Read the model definition and answer for the solid it produces. Units are mm, in the model's axes. Round coordinates to 2 decimals unless told otherwise and drop trailing zeros. Order: outer loops, then holes, each group sorted by start corner. A loop starts at its lowest first (then second) coordinate and runs counter-clockwise, first axis right, second up. Notation, with made-up numbers: (-33, -9.5) -> (22, -9.5) arc R22 ccw to (22, 14.5) -> close; hole circle Ø3 at (16, 17.25). An arc over 180 degrees is marked (long way). One line per item, written item: value. Start each with the question number.
1. Flat-ended cylindrical pins translate along their axes: pin 1 Ø1.5 at (x, y) = (-18.5, 1.5) entering from +Z; pin 2 Ø1 at (x, y) = (-9.5, 1.5) entering from -Z. Find the tip coordinate at first contact, or state that the pin passes through.
2. Section C-C (y = 1.55) is taken. Give the vertices of the cut face in (x, z).
3. Consider line 1 (Z direction, x = 0, y = 1.5); line 2 (Z direction, x = -11.5, y = 2.9); line 3 (X direction, y = 1.1, z = 6). Determine where each line is inside the solid, lowest interval first.
4. Section B-B (x = 0) is taken. Give the vertices of the cut face in (y, z), then the cut area to 3 significant figures.
5. Section A-A (z = 0) is taken. Give the vertices of the cut face in (x, y).
6. The mould has two halves that part along X. Classify faces 1 (the face through (12, 3, 6)), 2 (the face through (11.99, 1.51, 0.53)), 3 (the face through (13.38, 1.49, 25.73)): released by +X, released by -X, zero draft, split by the parting line, or undercut.
from build123d import *

# Parameters (mm, degrees)
SKETCH1_R          = 29
EXTRUDE1_DEPTH     = 3
SKETCH2_R          = 12
CUT_EXTRUDE1_DEPTH = 4
CHAMFER1_SIZE      = 0.5
CHAMFER2_SIZE      = 1


with BuildPart() as part:
    # Sketch1 → Extrude1 (new body)
    with BuildSketch(Plane(origin=(0, 0, 0), x_dir=(1, 0, 0), z_dir=(0, 1, 0))):
        Circle(SKETCH1_R)
    extrude(amount=EXTRUDE1_DEPTH)

    # Sketch2 → Cut-Extrude1 (cut, through all)
    with BuildSketch(Plane(origin=(0, 3, 0), x_dir=(-1, 0, 0), z_dir=(0, 1, 0))):
        Circle(SKETCH2_R)
    extrude(amount=-CUT_EXTRUDE1_DEPTH, mode=Mode.SUBTRACT)

    # Chamfer1
    chamfer1_edges = [part.edges().sort_by_distance(p)[0] for p in [
        (-29, 0, 0),
        (-29, 3, 0),
    ]]
    chamfer(chamfer1_edges, length=CHAMFER1_SIZE)

    # Chamfer2
    chamfer2_edges = [part.edges().sort_by_distance(p)[0] for p in [
        (12, 0, 0),
        (12, 3, 0),
    ]]
    chamfer(chamfer2_edges, length=CHAMFER2_SIZE)


solid = part.part
Answer:
1. pin 1: z = 22.93
1. pin 2: z = -27.57
2. outline: circle Ø58 at (0, 0); hole circle Ø24 at (0, 0)
3. line 1: -29 to -12, 12 to 29
3. line 2: -26.19 to -5.84, 5.84 to 26.19
3. line 3: -28.37 to -10.39, 10.39 to 28.37
4. outline: (0, -28.5) -> (0.5, -29) -> (2.5, -29) -> (3, -28.5) -> (3, -13) -> (2, -12) -> (1, -12) -> (0, -13) -> close; (0, 13) -> (1, 12) -> (2, 12) -> (3, 13) -> (3, 28.5) -> (2.5, 29) -> (0.5, 29) -> (0, 28.5) -> close
4. area: 99.5 mm^2
5. outline: (-29, 0.5) -> (-28.5, 0) -> (-13, 0) -> (-12, 1) -> (-12, 2) -> (-13, 3) -> (-28.5, 3) -> (-29, 2.5) -> close; (12, 1) -> (13, 0) -> (28.5, 0) -> (29, 0.5) -> (29, 2.5) -> (28.5, 3) -> (13, 3) -> (12, 2) -> close
6. face 1: zero draft
6. face 2: undercut
6. face 3: split by the parting line
